Can you work these out from the model? Positions are in its coordinate system, mm. Face numbers are marked on the shaded views. A direction names the side the tool comes from. Coordinates: 2 decimals unless noted, no trailing zeros. Write each loop counter-clockwise with the first axis right and the second up, starting at its lowest first coordinate (ties: lowest second). Pieces come first, ordered by that corner, then holes. Notation, with made-up numbers: (55.25, 17) -> (95.25, 17) arc R9 cw to (95.25, 22) -> close; hole circle Ø10 at (86.25, 32). An arc over 180 degrees is marked (long way). Answer as CSV lines item,"result". Start each with the question number.
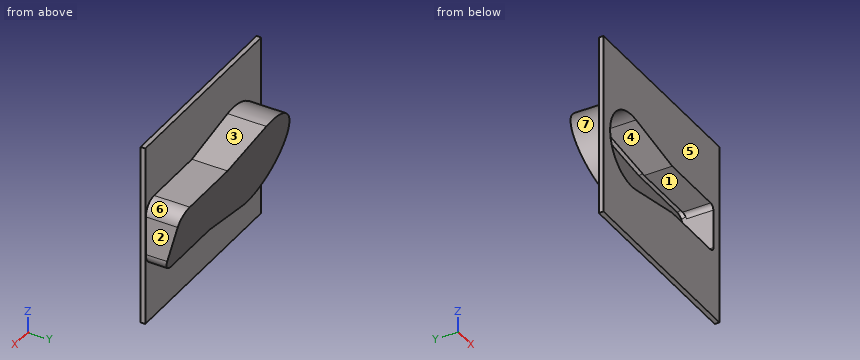
```python
from build123d import *

# Parameters (mm, degrees)
SKETCH_1_W          = 210
SKETCH_1_H          = 194
EXTRUDE_1_DEPTH     = 5
EXTRUDE_2_DEPTH     = 50
CUT_EXTRUDE_1_DEPTH = 292.137424595
FILLET_1_R          = 15
CUT_EXTRUDE_2_DEPTH = 15
CUT_EXTRUDE_4_DEPTH = 5
CUT_EXTRUDE_6_REACH = 289.625


with BuildPart() as part:
    # 草图1 → 凸台-拉伸1 (new body)
    with BuildSketch(Plane(origin=(0, 0, 0), x_dir=(1, 0, 0), z_dir=(0, 1, 0))):
        with Locations((105, -97)):
            Rectangle(SKETCH_1_W, SKETCH_1_H)
    extrude(amount=EXTRUDE_1_DEPTH)

    # 草图2 → 凸台-拉伸2 (add)
    with BuildSketch(Plane(origin=(0, 5, 0), x_dir=(1, 0, 0), z_dir=(0, 1, 0))):
        with BuildLine():
            Line((125.513628731, -61.215495335), (208.95, -61.215495335))
            Line((208.95, -61.215495335), (208.95, -132.784504665))
            Line((208.95, -132.784504665), (125.513628731, -132.784504665))
            Line((125.513628731, -132.784504665), (61.026324627, -145.513879526))
            ThreePointArc((61.026324627, -145.513879526), (2, -97), (61.026324627, -48.486120474))
            Line((61.026324627, -48.486120474), (125.513628731, -61.215495335))
        make_face()
    extrude(amount=EXTRUDE_2_DEPTH)

    # 草图3 → 切除-拉伸1 (cut, through all)
    with BuildSketch(Plane.ZY):
        Polygon((146.45, 46.500175131), (146.45, 55), (47.55, 55), (47.55, 20), align=None)
    extrude(amount=-CUT_EXTRUDE_1_DEPTH, mode=Mode.SUBTRACT)

    # 圆角1
    fillet_1_edges = [part.edges().sort_by_distance(p)[0] for p in [
        (208.95, 14.33082922, 61.215495335),
        (208.95, 23.919258346, 132.784504665),
    ]]
    fillet(fillet_1_edges, radius=FILLET_1_R)

    # 草图5 → 切除-拉伸2 (cut)
    with BuildSketch(Plane.XZ):
        with BuildLine():
            Line((124.536092452, 122.784504665), (59.089757463, 135.703185992))
            ThreePointArc((59.089757463, 135.703185992), (12, 97), (59.089757463, 58.296814008))
            Line((59.089757463, 58.296814008), (124.536092452, 71.215495335))
            Line((124.536092452, 71.215495335), (193.95, 71.215495335))
            ThreePointArc((193.95, 71.215495335), (197.485533906, 72.679961429), (198.95, 76.215495335))
            Line((198.95, 76.215495335), (198.95, 117.784504665))
            ThreePointArc((198.95, 117.784504665), (197.485533906, 121.320038571), (193.95, 122.784504665))
            Line((193.95, 122.784504665), (124.536092452, 122.784504665))
        make_face()
    extrude(amount=-CUT_EXTRUDE_2_DEPTH, mode=Mode.SUBTRACT)

    # 草图7 → 切除-拉伸4 (cut)
    with BuildSketch(Plane(origin=(0, 1.943124906, -0.520658749), x_dir=(1, 0, 0), z_dir=(0, 0.9659258262890681, -0.25881904510252174))):
        with BuildLine():
            Line((124.502295526, -129.347406371), (193.95, -129.347406371))
            add(Edge.make_bspline(
                [(193.95, -129.347406371), (194.562427767, -129.347406371), (195.774611757, -129.102068407), (197.439735395, -127.969946536), (198.650781168, -126.127504684), (198.95, -124.574413564), (198.95, -123.818263665)],
                knots=[-3.141592654, -3.141592654, -3.141592654, -3.141592654, -2.748893572, -2.35619449, -1.963495408, -1.570796327, -1.570796327, -1.570796327, -1.570796327], degree=3))
            Line((198.95, -123.818263665), (198.95, -80.782858462))
            add(Edge.make_bspline(
                [(198.95, -80.782858462), (198.95, -80.026708563), (198.650781168, -78.473617443), (197.439735395, -76.631175591), (195.774611757, -75.49905372), (194.562427767, -75.253715756), (193.95, -75.253715756)],
                knots=[-1.570796327, -1.570796327, -1.570796327, -1.570796327, -1.178097245, -0.785398163, -0.392699082, 0, 0, 0, 0], degree=3))
            Line((193.95, -75.253715756), (124.502295526, -75.253715756))
            Line((124.502295526, -75.253715756), (59.024136493, -61.872809237))
            add(Edge.make_bspline(
                [(59.024136493, -61.872809237), (56.210095744, -61.297740897), (50.427971911, -60.789688878), (38.964091843, -62.413259275), (25.731264842, -69.297623809), (14.654919531, -83.972220417), (10.672540234, -102.300561063), (14.654919531, -120.628901709), (25.731264842, -135.303498318), (38.964091843, -142.187862851), (50.427971911, -143.811433248), (56.210095744, -143.30338123), (59.024136493, -142.72831289)],
                knots=[-0.194888061, -0.194888061, -0.194888061, -0.194888061, 0.025822487, 0.246533036, 0.687954133, 1.12937523, 1.570796327, 2.012217424, 2.453638521, 2.895059618, 3.115770166, 3.336480715, 3.336480715, 3.336480715, 3.336480715], degree=3))
            Line((59.024136493, -142.72831289), (124.502295526, -129.347406371))
        make_face()
    extrude(amount=-CUT_EXTRUDE_4_DEPTH, mode=Mode.SUBTRACT)

    # 切除-拉伸6: up to this face of the body (flat: up to its plane)
    cut_extrude_6_end = Plane(part.part.faces().sort_by_distance((100.607454563, 28.420458434, 98.294095226))[0])
    # 草图8 → 切除-拉伸6 (cut, up to the picked face)
    with BuildSketch(Plane.XZ.offset(-15), mode=Mode.PRIVATE) as cut_extrude_6_sk1:
        with BuildLine():
            Line((193.95, 122.784504665), (124.536092452, 122.784504665))
            Line((124.536092452, 122.784504665), (59.089757463, 135.703185992))
            ThreePointArc((59.089757463, 135.703185992), (12, 97), (59.089757463, 58.296814008))
            Line((59.089757463, 58.296814008), (124.536092452, 71.215495335))
            Line((124.536092452, 71.215495335), (193.95, 71.215495335))
            ThreePointArc((193.95, 71.215495335), (197.485533906, 72.679961429), (198.95, 76.215495335))
            Line((198.95, 76.215495335), (198.95, 117.784504665))
            ThreePointArc((198.95, 117.784504665), (197.485533906, 121.320038571), (193.95, 122.784504665))
        make_face()
    cut_extrude_6_tool1 = split(extrude(cut_extrude_6_sk1.sketch, amount=-CUT_EXTRUDE_6_REACH, mode=Mode.PRIVATE), bisect_by=cut_extrude_6_end, keep=Keep.BOTH, mode=Mode.PRIVATE)
    add(cut_extrude_6_tool1.solids().sort_by(Axis((100.513282, 15, 97), (0, 1, 0)))[0], mode=Mode.SUBTRACT)


solid = part.part
```
Q1. For pin 1 (6 mm diameter, centred on x = 128, z = 91.5, fed in from +Y); pin 2 (11.5 mm diameter, centred on x = 160, y = 18, fed in from +Z); pin 3 (9.5 mm diameter, centred on x = 150, y = 15, fed in from -Z), each with a flat end and sliding along its axis, tell me the tip position at first contact or that it passes through.
Q2. I need wall thicknesses on L1, parallel to Z at x = 51.45, y = 16.5; L2, parallel to X at y = 8, z = 97; L3, parallel to Z at x = 186.5, y = 11.5. Which ranges of each line are inside material? Lowest first, please.
Q3. Imagine slicing it at B-B (x = 133.5). Write out the boundary of the cut face in (y, z).
Q4. Imagine slicing it at D-D (x = 83). Write out the boundary of the cut face in (y, z).
Q5. Which directions (+Z, -Z, +X, -X, +Y, -Y) give clear straight access to the entire face, cutting with the end or side of a thin tool? Please do the marked faces 4, 5, 6 and 7.
Q6. Imagine slicing it at C-C (z = 52.5). Write out the boundary of the cut face in (x, y).
Q7. If we mould it in two halves opening along Z, with no side actions, what happens to the marked faces 1, 2 and 3? For each: released by +Z, released by -Z, zero draft, split by the parting line, or undercut.
Q8. Imagine slicing it at A-A (y = 11). Write out the boundary of the cut face in (x, z).
Entries:
1,pin 1,"y = 32.58"
1,pin 2,"z = 132.78"
1,pin 3,"z = 61.22"
2,L1,"47.55 to 57.55, 136.45 to 146.45"
2,L2,"2 to 12, 198.95 to 208.95"
2,L3,"61.22 to 71.22, 122.78 to 132.78"
3,outline,"(0, 0) -> (5, 0) -> (5, 61.22) -> (23.66, 61.22) -> (42.84, 132.78) -> (5, 132.78) -> (5, 194) -> (0, 194) -> (0, 122.78) -> (29.81, 122.78) -> (30.59, 125.71) -> (35.42, 124.42) -> (21.16, 71.22) -> (0, 71.22) -> close"
4,outline,"(0, 0) -> (5, 0) -> (5, 52.82) -> (21.41, 52.82) -> (45.09, 141.18) -> (5, 141.18) -> (5, 194) -> (0, 194) -> (0, 130.98) -> (32, 130.98) -> (32.79, 133.91) -> (37.62, 132.61) -> (18.97, 63.02) -> (0, 63.02) -> close"
5,face 4,"-Y"
5,face 5,"+Z, -Z, +X, -X, -Y"
5,face 6,"+Z, +X, +Y"
5,face 7,"+Y"
6,outline,"(0, 0) -> (210, 0) -> (210, 5) -> (81.36, 5) -> (81.36, 21.33) -> (29.88, 21.33) -> (29.88, 5) -> (0, 5) -> close"
7,face 1,"undercut"
7,face 2,"zero draft"
7,face 3,"released by +Z"
8,outline,"(61.03, 48.49) -> (125.51, 61.22) -> (193.95, 61.22) arc R15 ccw to (208.95, 76.22) -> (208.95, 117.78) arc R15 ccw to (193.95, 132.78) -> (125.51, 132.78) -> (61.03, 145.51) arc R49.45 ccw (long way) to start; hole (59.09, 58.3) -> (124.54, 71.22) -> (193.95, 71.22) arc R5 ccw to (198.95, 76.22) -> (198.95, 117.78) arc R5 ccw to (193.95, 122.78) -> (124.54, 122.78) -> (59.09, 135.7) arc R39.45 ccw (long way) to start"
